Design review of the part built by this model. Coordinates are the model's own, in mm. A direction names the side the tool comes from. Round coordinates to 2 decimals unless told otherwise and drop trailing zeros. Loops run counter-clockwise (first coordinate to the right, second up) from the corner with the lowest first, then second, coordinate; pieces in that order, holes last. Notation, with made-up numbers: M -10,-23.5 L 1,-23.5 A13 cw 1,-2.5 Z; hole C 2,-32 d7. An arc over 180 degrees is marked long. One line per item, written item: value. Start each with the question number.
Item 1: Mouldability with a two-part tool opening along Y and no side actions: class faces 4 (the cylindrical face through (26.045, 24.385, 52.614)), 5 (the cylindrical face through (-0.69, -3.1, 65.91)), 6 (the cylindrical face through (-25.638, -25.168, 52.614)), 7 (the cylindrical face through (17.078, 27.216, 24.669)) as released by +Y, released by -Y, zero draft, split by the parting line, or undercut.
Item 2: We need section C-C (z = 53). Write out the cut boundary in (x, y) (3 decimals).
Item 3: For faces 1 (the cylindrical face through (17.01, -27.26, 24.67)), 2 (the cylindrical face through (27.26, 17.01, 24.67)), 3 (the flat face through (-19.279, 24, 25)), list the 3-axis set-ups (+Z, -Z, +X, -X, +Y, -Y) from which the entire face can be reached by the end or side of a thin tool; tool diameter is ignored.
Item 4: We need section A-A (y = 0). Write out the cut boundary in (x, z) (3 decimals), then the cut area to 3 significant figures.
Item 5: Clearance check with flat-ended pins moving along their axes: pin 1 (4.5 mm diameter, centred on x = -23, z = 19.5, fed in from +Y); pin 2 (4.5 mm diameter, centred on y = -24.5, z = 16.5, fed in from +X); pin 3 (3 mm diameter, centred on x = 3.5, z = 51, fed in from +Y) (3 decimals). State where each tip first meets the part, or that it passes through.
Item 6: We need section D-D (y = 52.5). Write out the cut boundary in (x, z) (3 decimals).
Item 7: We need section B-B (z = 28). Write out the cut boundary in (x, y) (3 decimals).
Item 8: For line 1 along Y through (x, z) = (0, 51) (3 decimals); line 2 along Y through (x, z) = (23.5, 28); line 3 along Z through (x, y) = (5.5, -4), list the stretches that pass through material, from the lowest coordinate up.
from build123d import *

# Parameters (mm, degrees)
SKETCH1_W           = 57.15
SKETCH1_H           = 57.15
BOSS_EXTRUDE1_DEPTH = 55.118
CUT_EXTRUDE1_DEPTH  = 50.038
CUT_EXTRUDE2_DEPTH  = 50.038
CUT_EXTRUDE3_DEPTH  = 50.038
CUT_EXTRUDE4_DEPTH  = 50.038
CUT_EXTRUDE5_DEPTH  = 50.038
CUT_EXTRUDE6_DEPTH  = 50.038
CUT_EXTRUDE7_DEPTH  = 50.038
CUT_EXTRUDE8_DEPTH  = 50.038
SKETCH10_R          = 19.05
BOSS_EXTRUDE2_DEPTH = 1.524
SKETCH11_R          = 3.175
BOSS_EXTRUDE3_DEPTH = 19.05
CUT_EXTRUDE9_DEPTH  = 14.986
SKETCH13_W          = 0.635
SKETCH13_H          = 85.725
SKETCH14_W          = 0.635
SKETCH14_H          = 85.725
SKETCH15_W          = 0.635
SKETCH15_H          = 85.725
SKETCH16_W          = 0.635
SKETCH16_H          = 85.725
HOLE1_D             = 5.08
HOLE1_DEPTH         = 25.654
HOLE2_D             = 5.08
HOLE2_DEPTH         = 25.654
HOLE3_D             = 5.08
HOLE3_DEPTH         = 25.654
HOLE4_D             = 5.08
HOLE4_DEPTH         = 25.654
CHAMFER1_SIZE       = 0.254
FILLET1_R           = 2.54
FILLET2_R           = 2.54
FILLET3_R           = 2.54
FILLET4_R           = 2.54
FILLET5_R           = 2.54
FILLET6_R           = 2.54
FILLET7_R           = 2.54
FILLET8_R           = 2.54


with BuildPart() as part:
    # Sketch1 → Boss-Extrude1 (new body)
    with BuildSketch(Plane.XY.offset(55.118)):
        Rectangle(SKETCH1_W, SKETCH1_H)
    extrude(amount=-BOSS_EXTRUDE1_DEPTH)

    # Sketch2 → Cut-Extrude1 (cut)
    with BuildSketch(Plane(origin=(0, 0, 0), x_dir=(-1, 0, 0), z_dir=(0, 0, -1))):
        with BuildLine():
            Line((-28.575, -28.575), (-14.692533342, -28.575))
            ThreePointArc((-14.692533342, -28.575), (-22.720047986, -22.720047986), (-28.575, -14.692533342))
            Line((-28.575, -14.692533342), (-28.575, -28.575))
        make_face()
    extrude(amount=-CUT_EXTRUDE1_DEPTH, mode=Mode.SUBTRACT)

    # Sketch3 → Cut-Extrude2 (cut)
    with BuildSketch(Plane(origin=(0, 0, 0), x_dir=(-1, 0, 0), z_dir=(0, 0, -1))):
        with BuildLine():
            Line((-19.2786, -25.7048), (-19.2786, -19.2786))
            Line((-19.2786, -19.2786), (-25.7048, -19.2786))
            ThreePointArc((-25.7048, -19.2786), (-22.720047986, -22.720047986), (-19.2786, -25.7048))
        make_face()
    extrude(amount=-CUT_EXTRUDE2_DEPTH, mode=Mode.SUBTRACT)

    # Sketch4 → Cut-Extrude3 (cut)
    with BuildSketch(Plane(origin=(0, 0, 0), x_dir=(-1, 0, 0), z_dir=(0, 0, -1))):
        with BuildLine():
            Line((-28.575, 28.575), (-28.575, 14.692533342))
            ThreePointArc((-28.575, 14.692533342), (-22.720047986, 22.720047986), (-14.692533342, 28.575))
            Line((-14.692533342, 28.575), (-28.575, 28.575))
        make_face()
    extrude(amount=-CUT_EXTRUDE3_DEPTH, mode=Mode.SUBTRACT)

    # Sketch5 → Cut-Extrude4 (cut)
    with BuildSketch(Plane(origin=(0, 0, 0), x_dir=(-1, 0, 0), z_dir=(0, 0, -1))):
        with BuildLine():
            Line((-25.7048, 19.2786), (-19.2786, 19.2786))
            Line((-19.2786, 19.2786), (-19.2786, 25.7048))
            ThreePointArc((-19.2786, 25.7048), (-22.720047986, 22.720047986), (-25.7048, 19.2786))
        make_face()
    extrude(amount=-CUT_EXTRUDE4_DEPTH, mode=Mode.SUBTRACT)

    # Sketch6 → Cut-Extrude5 (cut)
    with BuildSketch(Plane(origin=(0, 0, 0), x_dir=(-1, 0, 0), z_dir=(0, 0, -1))):
        with BuildLine():
            Line((28.575, 28.575), (14.692533342, 28.575))
            ThreePointArc((14.692533342, 28.575), (22.720047986, 22.720047986), (28.575, 14.692533342))
            Line((28.575, 14.692533342), (28.575, 28.575))
        make_face()
    extrude(amount=-CUT_EXTRUDE5_DEPTH, mode=Mode.SUBTRACT)

    # Sketch7 → Cut-Extrude6 (cut)
    with BuildSketch(Plane(origin=(0, 0, 0), x_dir=(-1, 0, 0), z_dir=(0, 0, -1))):
        with BuildLine():
            Line((19.2786, 25.7048), (19.2786, 19.2786))
            Line((19.2786, 19.2786), (25.7048, 19.2786))
            ThreePointArc((25.7048, 19.2786), (22.720047986, 22.720047986), (19.2786, 25.7048))
        make_face()
    extrude(amount=-CUT_EXTRUDE6_DEPTH, mode=Mode.SUBTRACT)

    # Sketch8 → Cut-Extrude7 (cut)
    with BuildSketch(Plane(origin=(0, 0, 0), x_dir=(-1, 0, 0), z_dir=(0, 0, -1))):
        with BuildLine():
            Line((28.575, -28.575), (28.575, -14.692533342))
            ThreePointArc((28.575, -14.692533342), (22.720047986, -22.720047986), (14.692533342, -28.575))
            Line((14.692533342, -28.575), (28.575, -28.575))
        make_face()
    extrude(amount=-CUT_EXTRUDE7_DEPTH, mode=Mode.SUBTRACT)

    # Sketch9 → Cut-Extrude8 (cut)
    with BuildSketch(Plane(origin=(0, 0, 0), x_dir=(-1, 0, 0), z_dir=(0, 0, -1))):
        with BuildLine():
            Line((25.7048, -19.2786), (19.2786, -19.2786))
            Line((19.2786, -19.2786), (19.2786, -25.7048))
            ThreePointArc((19.2786, -25.7048), (22.720047986, -22.720047986), (25.7048, -19.2786))
        make_face()
    extrude(amount=-CUT_EXTRUDE8_DEPTH, mode=Mode.SUBTRACT)

    # Sketch10 → Boss-Extrude2 (add)
    with BuildSketch(Plane.XY.offset(55.118)):
        Circle(SKETCH10_R)
    extrude(amount=BOSS_EXTRUDE2_DEPTH)

    # Sketch11 → Boss-Extrude3 (add)
    with BuildSketch(Plane.XY.offset(56.642)):
        Circle(SKETCH11_R)
    extrude(amount=BOSS_EXTRUDE3_DEPTH)

    # Sketch12 → Cut-Extrude9 (cut)
    with BuildSketch(Plane.XY.offset(75.692)):
        with BuildLine():
            Line((-1.722711816, 2.667), (1.722711816, 2.667))
            ThreePointArc((1.722711816, 2.667), (0, 3.175), (-1.722711816, 2.667))
        make_face()
    extrude(amount=-CUT_EXTRUDE9_DEPTH, mode=Mode.SUBTRACT)

    # Sketch13 → Revolve1 (revolve)
    with BuildSketch(Plane(origin=(0, 0, 12.7), x_dir=(-1, 0, 0), z_dir=(0, 0, -1))):
        with Locations((1.7145, 71.4375)):
            Rectangle(SKETCH13_W, SKETCH13_H)
    revolve(axis=Axis((-2.032, 28.575, 12.7), (0, 1, 0)))

    # Sketch14 → Revolve2 (revolve)
    with BuildSketch(Plane(origin=(0, 0, 12.7), x_dir=(-1, 0, 0), z_dir=(0, 0, -1))):
        with Locations((-2.3495, 71.4375)):
            Rectangle(SKETCH14_W, SKETCH14_H)
    revolve(axis=Axis((2.032, 28.575, 12.7), (0, 1, 0)))

    # Sketch15 → Revolve3 (revolve)
    with BuildSketch(Plane(origin=(0, 0, 14.732), x_dir=(-1, 0, 0), z_dir=(0, 0, -1))):
        with Locations((-0.3175, 71.4375)):
            Rectangle(SKETCH15_W, SKETCH15_H)
    revolve(axis=Axis((0, 28.575, 14.732), (0, 1, 0)))

    # Sketch16 → Revolve4 (revolve)
    with BuildSketch(Plane(origin=(0, 0, 10.668), x_dir=(-1, 0, 0), z_dir=(0, 0, -1))):
        with Locations((-0.3175, 71.4375)):
            Rectangle(SKETCH16_W, SKETCH16_H)
    revolve(axis=Axis((0, 28.575, 10.668), (0, 1, 0)))

    # Hole1
    with Locations(Plane(origin=(0, 0, 50.038), x_dir=(-1, 0, 0), z_dir=(0, 0, -1))):
        with Locations((23.622, -23.622)):
            Hole(HOLE1_D / 2, depth=HOLE1_DEPTH)

    # Hole2
    with Locations(Plane(origin=(0, 0, 50.038), x_dir=(-1, 0, 0), z_dir=(0, 0, -1))):
        with Locations((23.622, 23.622)):
            Hole(HOLE2_D / 2, depth=HOLE2_DEPTH)

    # Hole3
    with Locations(Plane(origin=(0, 0, 50.038), x_dir=(-1, 0, 0), z_dir=(0, 0, -1))):
        with Locations((-23.622, 23.622)):
            Hole(HOLE3_D / 2, depth=HOLE3_DEPTH)

    # Hole4
    with Locations(Plane(origin=(0, 0, 50.038), x_dir=(-1, 0, 0), z_dir=(0, 0, -1))):
        with Locations((-23.622, -23.622)):
            Hole(HOLE4_D / 2, depth=HOLE4_DEPTH)

    # Chamfer1
    chamfer1_edges = [part.edges().sort_by_distance(p)[0] for p in [
        (-1.51838977, -2.78838977, 75.692),
    ]]
    chamfer(chamfer1_edges, length=CHAMFER1_SIZE)

    # Fillet1
    fillet1_edges = [part.edges().sort_by_distance(p)[0] for p in [
        (-28.575, 28.575, 52.578),
    ]]
    fillet(fillet1_edges, radius=FILLET1_R)

    # Fillet2
    fillet2_edges = [part.edges().sort_by_distance(p)[0] for p in [
        (-28.575, -28.575, 52.578),
    ]]
    fillet(fillet2_edges, radius=FILLET2_R)

    # Fillet3
    fillet3_edges = [part.edges().sort_by_distance(p)[0] for p in [
        (28.575, 28.575, 52.578),
    ]]
    fillet(fillet3_edges, radius=FILLET3_R)

    # Fillet4
    fillet4_edges = [part.edges().sort_by_distance(p)[0] for p in [
        (-19.2786, 19.2786, 25.019),
    ]]
    fillet(fillet4_edges, radius=FILLET4_R)

    # Fillet5
    fillet5_edges = [part.edges().sort_by_distance(p)[0] for p in [
        (28.575, -28.575, 52.578),
    ]]
    fillet(fillet5_edges, radius=FILLET5_R)

    # Fillet6
    fillet6_edges = [part.edges().sort_by_distance(p)[0] for p in [
        (19.2786, -19.2786, 25.019),
    ]]
    fillet(fillet6_edges, radius=FILLET6_R)

    # Fillet7
    fillet7_edges = [part.edges().sort_by_distance(p)[0] for p in [
        (19.2786, 19.2786, 25.019),
    ]]
    fillet(fillet7_edges, radius=FILLET7_R)

    # Fillet8
    fillet8_edges = [part.edges().sort_by_distance(p)[0] for p in [
        (-19.2786, -19.2786, 25.019),
    ]]
    fillet(fillet8_edges, radius=FILLET8_R)


solid = part.part
A:
1. face 4: undercut
1. face 5: split by the parting line
1. face 6: undercut
1. face 7: released by +Y
2. outline: M -28.575,-26.035 A2.54 ccw -26.035,-28.575 L 26.035,-28.575 A2.54 ccw 28.575,-26.035 L 28.575,26.035 A2.54 ccw 26.035,28.575 L -26.035,28.575 A2.54 ccw -28.575,26.035 Z; hole C -23.622,-23.622 d5.08; hole C -23.622,23.622 d5.08; hole C 23.622,-23.622 d5.08; hole C 23.622,23.622 d5.08
3. face 1: -Z, +X, -Y
3. face 2: -Z, +X, +Y
3. face 3: -Z, -X, +Y
4. outline: M -28.575,0 L 28.575,0 L 28.575,55.118 L 19.05,55.118 L 19.05,56.642 L 3.175,56.642 L 3.175,75.438 L 2.921,75.692 L -2.921,75.692 L -3.175,75.438 L -3.175,56.642 L -19.05,56.642 L -19.05,55.118 L -28.575,55.118 Z
4. area: 3,330 mm2
5. pin 1: y = 19.51
5. pin 2: x = 19.28
5. pin 3: y = 28.575
6. outline: C -2.032,12.7 d1.27; C 0,10.668 d1.27; C 0,14.732 d1.27; C 2.032,12.7 d1.27
7. outline: M -28.575,-14.693 A32.131 ccw -25.705,-19.279 L -21.819,-19.279 A2.54 cw -19.279,-21.819 L -19.279,-25.705 A32.131 ccw -14.693,-28.575 L 14.693,-28.575 A32.131 ccw 19.279,-25.705 L 19.279,-21.819 A2.54 cw 21.819,-19.279 L 25.705,-19.279 A32.131 ccw 28.575,-14.693 L 28.575,14.693 A32.131 ccw 25.705,19.279 L 21.819,19.279 A2.54 cw 19.279,21.819 L 19.279,25.705 A32.131 ccw 14.693,28.575 L -14.693,28.575 A32.131 ccw -19.279,25.705 L -19.279,21.819 A2.54 cw -21.819,19.279 L -25.705,19.279 A32.131 ccw -28.575,14.693 Z
8. line 1: -28.575 to 28.575
8. line 2: -19.28 to 19.28
8. line 3: 0 to 56.64
